```python
from build123d import *

# Parameters (mm, degrees)
F0_R      = 6
F1_DEPTH  = 40
F3_DEPTH  = 15
F6_SIZE   = 0.5
F8_DEPTH  = 16.0010001
F9_R      = 1.25
F10_DEPTH = 4.1326528028
F11_DEPTH = 15


# Not quite as in the source:
# - a feature names something its author has since deleted; it is built from what else it names


with BuildPart() as f1:
    # F0 (on Top) → F1 (new body)
    with BuildSketch(Plane.XY):
        with BuildLine():
            Line((-8, 6.1231056256), (-8, -2.1231056256))
            ThreePointArc((-8, -2.1231056256), (0, -7), (8, -2.1231056256))
            Line((8, -2.1231056256), (8, 6.1231056256))
            ThreePointArc((8, 6.1231056256), (6.1160859286, 8.6025368544), (3.5, 10.2915619759))
            Line((3.5, 10.2915619759), (3.5, 10))
            Line((3.5, 10), (-3.5, 10))
            Line((-3.5, 10), (-3.5, 10.2915619759))
            ThreePointArc((-3.5, 10.2915619759), (-6.1160859286, 8.6025368544), (-8, 6.1231056256))
        make_face()
        Circle(F0_R, mode=Mode.SUBTRACT)
    extrude(amount=F1_DEPTH)

    # F2 (on face) → F3 (cut)
    with BuildSketch(Plane.XY.offset(40)):
        with BuildLine():
            ThreePointArc((5.1812656518, -4.7068552395), (6.5295045586, -2.5230081686), (7, 0))
            ThreePointArc((7, 0), (-2.8330207662, 6.4010931362), (-4.7068552395, -5.1812656518))
            Line((-4.7068552395, -5.1812656518), (-4.0344473482, -4.4410848444))
            ThreePointArc((-4.0344473482, -4.4410848444), (-2.4283035139, 5.4866512596), (6, 0))
            ThreePointArc((6, 0), (5.5967181931, -2.1625784302), (4.4410848444, -4.0344473482))
            Line((4.4410848444, -4.0344473482), (5.1812656518, -4.7068552395))
        make_face()
        with BuildLine():
            Line((-4.0344473482, -4.4410848444), (-4.7068552395, -5.1812656518))
            ThreePointArc((-4.7068552395, -5.1812656518), (-2.523008134, -6.529504572), (7.42e-08, -7))
            ThreePointArc((7.42e-08, -7), (2.8330208001, -6.4010931212), (5.1812656518, -4.7068552395))
            Line((5.1812656518, -4.7068552395), (4.4410848444, -4.0344473482))
            ThreePointArc((4.4410848444, -4.0344473482), (0.2875361311, -5.9931062875), (-4.0344473482, -4.4410848444))
        make_face()
        with BuildLine():
            ThreePointArc((7.42e-08, -7), (-2.523008134, -6.529504572), (-4.7068552395, -5.1812656518))
            Line((-4.7068552395, -5.1812656518), (-4.9883233954, -5.4911033702))
            ThreePointArc((-4.9883233954, -5.4911033702), (-2.6057694927, -6.6145206106), (7.42e-08, -7))
        make_face()
        with BuildLine():
            Line((5.5754867215, -5.0649803835), (5.1812656518, -4.7068552395))
            ThreePointArc((5.1812656518, -4.7068552395), (2.8330208001, -6.4010931212), (7.42e-08, -7))
            ThreePointArc((7.42e-08, -7), (2.9508623284, -6.5024944292), (5.5754867215, -5.0649803835))
        make_face()
    extrude(amount=-F3_DEPTH, mode=Mode.SUBTRACT)

    # F4 (on Front) → F5 (revolve, cut)
    with BuildSketch(Plane.XZ):
        Polygon((0, 44.0566428006), (8, 40), (14.6664504582, 28.4533691002), (14.6664504582, 47.2484640777), (0, 47.2484640777), align=None)
    revolve(axis=Axis((0, 0, 27), (0, 0, 1)), mode=Mode.SUBTRACT)

    # F6
    f6_edges = [f1.edges().sort_by_distance(p)[0] for p in [
        (6.116086, 8.602537, 0),
        (-6.116086, 8.602537, 0),
        (-8, 2, 0),
        (0, -7, 0),
        (8, 2, 0),
    ]]
    chamfer(f6_edges, length=F6_SIZE)

    # F7 (on face) → F8 (cut, through all)
    with BuildSketch(Plane(origin=(-8, 0, 0), x_dir=(0, -1, 0), z_dir=(-1, 0, 0))):
        with BuildLine():
            ThreePointArc((2.1231056256, 5.6099524336), (3.4994587083, 7.0625303231), (4, 9))
            ThreePointArc((4, 9), (3.7742546282, 10.3247648854), (3.1224989992, 11.5))
            ThreePointArc((3.1224989992, 11.5), (2.6602891079, 11.0128840226), (2.1231056256, 10.6099524336))
            Line((2.1231056256, 10.6099524336), (2.1231056256, 5.6099524336))
        make_face()
        with BuildLine():
            ThreePointArc((3.1224989992, 11.5), (3.7742546282, 10.3247648854), (4, 9))
            Line((4, 9), (4, 14))
            ThreePointArc((4, 14), (3.7742546282, 12.6752351146), (3.1224989992, 11.5))
        make_face()
        with BuildLine():
            ThreePointArc((2.1231056256, 10.6099524336), (2.6602891079, 11.0128840226), (3.1224989992, 11.5))
            ThreePointArc((3.1224989992, 11.5), (2.6602891079, 11.9871159774), (2.1231056256, 12.3900475664))
            Line((2.1231056256, 12.3900475664), (2.1231056256, 10.6099524336))
        make_face()
        with BuildLine():
            ThreePointArc((2.1231056256, 12.3900475664), (2.6602891079, 11.9871159774), (3.1224989992, 11.5))
            ThreePointArc((3.1224989992, 11.5), (3.7742546282, 12.6752351146), (4, 14))
            ThreePointArc((4, 14), (3.4994587083, 15.9374696769), (2.1231056256, 17.3900475664))
            Line((2.1231056256, 17.3900475664), (2.1231056256, 12.3900475664))
        make_face()
        with BuildLine():
            ThreePointArc((-4, 9), (-1.9374696769, 5.5005412917), (2.1231056256, 5.6099524336))
            Line((2.1231056256, 5.6099524336), (2.1231056256, 10.6099524336))
            ThreePointArc((2.1231056256, 10.6099524336), (-0.66913597, 10.0563649949), (-3.1224989992, 11.5))
            ThreePointArc((-3.1224989992, 11.5), (-3.7742546282, 10.3247648854), (-4, 9))
        make_face()
        with BuildLine():
            Line((2.1231056256, 10.6099524336), (2.1231056256, 12.3900475664))
            ThreePointArc((2.1231056256, 12.3900475664), (-0.66913597, 12.9436350051), (-3.1224989992, 11.5))
            ThreePointArc((-3.1224989992, 11.5), (-0.66913597, 10.0563649949), (2.1231056256, 10.6099524336))
        make_face()
        with BuildLine():
            ThreePointArc((-3.1224989992, 11.5), (-0.66913597, 12.9436350051), (2.1231056256, 12.3900475664))
            Line((2.1231056256, 12.3900475664), (2.1231056256, 17.3900475664))
            ThreePointArc((2.1231056256, 17.3900475664), (-1.9374696769, 17.4994587083), (-4, 14))
            ThreePointArc((-4, 14), (-3.7742546282, 12.6752351146), (-3.1224989992, 11.5))
        make_face()
        with BuildLine():
            Line((-4, 14), (-4, 9))
            ThreePointArc((-4, 9), (-3.7742546282, 10.3247648854), (-3.1224989992, 11.5))
            ThreePointArc((-3.1224989992, 11.5), (-3.7742546282, 12.6752351146), (-4, 14))
        make_face()
    extrude(amount=-F8_DEPTH, mode=Mode.SUBTRACT)

    # F9 (on face) → F10 (cut, through all)
    with BuildSketch(Plane(origin=(0, 10, 0), x_dir=(-1, 0, 0), z_dir=(0, 1, 0))):
        with Locations((0, 3.5)):
            Circle(F9_R)
        with Locations((0, 22)):
            Circle(F9_R)
        with Locations((0, 27)):
            Circle(F9_R)
        with Locations((0, 32)):
            Circle(F9_R)
    extrude(amount=-F10_DEPTH, mode=Mode.SUBTRACT)

    # F9 (on face) → F11 (cut)
    with BuildSketch(Plane(origin=(0, 10, 0), x_dir=(-1, 0, 0), z_dir=(0, 1, 0))):
        with BuildLine():
            ThreePointArc((-6.5, 18), (-7.232233047, 19.767766953), (-9, 20.5))
            Line((-9, 20.5), (-9.5, 20.5))
            Line((-9.5, 20.5), (-9.5, 2.5))
            Line((-9.5, 2.5), (-9, 2.5))
            ThreePointArc((-9, 2.5), (-7.232233047, 3.232233047), (-6.5, 5))
            Line((-6.5, 5), (-6.5, 18))
        make_face()
        with BuildLine():
            Line((10.5, 20.5), (9, 20.5))
            ThreePointArc((9, 20.5), (7.232233047, 19.767766953), (6.5, 18))
            Line((6.5, 18), (6.5, 5))
            ThreePointArc((6.5, 5), (7.232233047, 3.232233047), (9, 2.5))
            Line((9, 2.5), (10.5, 2.5))
            Line((10.5, 2.5), (10.5, 20.5))
        make_face()
    extrude(amount=-F11_DEPTH, mode=Mode.SUBTRACT)


solid = f1.part
```
Design review of the part built by this model. Coordinates are the model's own, in mm. A direction names the side the tool comes from. Give positions to 0.01 mm unless a question says otherwise; leave off trailing zeros. Write each loop counter-clockwise with the first axis right and the second up, starting at its lowest first coordinate (ties: lowest second). Pieces come first, ordered by that corner, then holes. Notation, with made-up numbers: (51.25, -34) - (87.25, -34) arc R17 cw to (87.25, -10) - close; hole circle Ø1 at (-28.5, 50.5). An arc over 180 degrees is marked (long way). Return JSON: item names as keys, results as strings. Group by question number.
(1) Machinability: for faces 4 (the flat face through (-6, -4, 11)), 5 (the flat face through (0, 10, 18)), 6 (the flat face through (-6.5, 6, 12)), which of the approach directions +Z, -Z, +X, -X, +Y, -Y give a long, thin tool a straight path to every point of the face, cutting with its end or side? Answer none if there is none.
(2) To check wall thickness, follow probe 1 along Z at (x, y) = (0, 8.7); probe 2 along Z at (x, y) = (0, 8.15); probe 3 along Y at (x, z) = (0, 28.75). State the ranges of each line that lie inside material, in increasing order.
(3) We need section C-C, the plane z = 24. Give the boundary of the cut face in (x, y), then the cut area to 3 significant figures.
(4) We need section B-B, the plane x = 0. Give the boundary of the cut face in (y, z), then the cut area to 3 significant figures.
(5) We need section D-D, the plane z = 3.5. Give the boundary of the cut face in (x, y).
(6) Insertion check: pin 1 (2 mm diameter, centred on x = -5.5, z = 12, fed in from -Y); pin 2 (3 mm diameter, centred on x = 0, z = 32, fed in from +Y); pin 3 (0.6 mm diameter, centred on x = -6, z = 12.5, fed in from +Y). Each pin has a flat end and moves straight along its axis. Give the tip position at first contact, or say it passes through.
(7) Mouldability with a two-part tool opening along X and no side actions: class faces 1 (the flat face through (8, 2, 2)), 2 (the flat face through (-8, 2, 2)), 3 (the flat face through (-2, -6, 25)) as +X half, -X half, draft (parallel to the pull), parting line (faces both ways), or undercut.
(8) We need section A-A, the plane z = 13. Give the boundary of the cut face in (x, y), then the cut area to 3 significant figures.
Reported:
{
 "1": {"face 4": "+X, -X", "face 5": "+Z, -Z, +Y", "face 6": "-X, +Y, -Y"},
 "2": {"probe 1": "z = 0 to 2.25, 4.75 to 20.75, 23.25 to 25.75, 28.25 to 30.75, 33.25 to 38.79", "probe 2": "z = 0 to 2.25, 4.75 to 20.75, 23.25 to 25.75, 28.25 to 30.75, 33.25 to 39.74", "probe 3": "y = 7 to 10"},
 "3": {"outline": "(-8, -2.12) arc R9 ccw to (8, -2.12) - (8, 6.12) arc R9 ccw to (3.5, 10.29) - (3.5, 10) - (-3.5, 10) - (-3.5, 10.29) arc R9 ccw to (-8, 6.12) - close; hole circle Ø12 at (0, 0)", "area": "125 mm2"},
 "4": {"outline": "(-7, 0.5) - (-6.5, 0) - (-6, 0) - (-6, 25) - (-7, 25) - close; (6, 0) - (10, 0) - (10, 2.25) - (6, 2.25) - close; (6, 4.75) - (10, 4.75) - (10, 20.75) - (6, 20.75) - close; (6, 23.25) - (10, 23.25) - (10, 25.75) - (7, 25.75) - (7, 25) - (6, 25) - close; (7, 28.25) - (10, 28.25) - (10, 30.75) - (7, 30.75) - close; (7, 33.25) - (10, 33.25) - (10, 36.54) - (8, 40) - (7, 40) - close", "area": "131 mm2"},
 "5": {"outline": "(-7, -3.66) arc R9 ccw to (7, -3.66) - (7, 7.66) arc R9 ccw to (3.5, 10.29) - (3.5, 10) - (1.25, 10) - (1.25, 5.87) arc R6 cw (long way) to (-1.25, 5.87) - (-1.25, 10) - (-3.5, 10) - (-3.5, 10.29) arc R9 ccw to (-7, 7.66) - close"},
 "6": {"pin 1": "stops at y = -5.79", "pin 2": "stops at y = 10", "pin 3": "stops at y = 8.96"},
 "7": {"face 1": "+X half", "face 2": "-X half", "face 3": "undercut"},
 "8": {"outline": "(-6.5, -4.22) arc R9 ccw to (6.5, -4.22) - (6.5, -4) - (4.47, -4) arc R6 cw to (-4.47, -4) - (-6.5, -4) - close; (-6.5, 4) - (-4.47, 4) arc R6 cw to (4.47, 4) - (6.5, 4) - (6.5, 8.22) arc R9 ccw to (3.5, 10.29) - (3.5, 10) - (-3.5, 10) - (-3.5, 10.29) arc R9 ccw to (-6.5, 8.22) - close", "area": "77.5 mm2"}
}
